from build123d import *

# Parameters (mm, degrees)
F0_W     = 762
F0_H     = 152.4
F1_DEPTH = 304.8
F2_T     = -25.4
F3_R     = 25.4
F4_DEPTH = 381
F5_R     = 12.7


with BuildPart() as f1:
    # F0 (on Front) → F1 (new body, symmetric)
    with BuildSketch(Plane.XZ):
        with Locations((0, 457.2)):
            Rectangle(F0_W, F0_H)
    extrude(amount=F1_DEPTH, both=True)

    # F2
    f2_openings = [f1.faces().sort_by_distance(p)[0] for p in [
        (0, -304.8, 457.2),
    ]]
    offset(amount=F2_T, openings=f2_openings)

    # F3 (on Top) → F4 (join, symmetric)
    with BuildSketch(Plane.XY):
        with Locations((-355.6, 279.4)):
            Circle(F3_R)
        with Locations((355.6, 279.4)):
            Circle(F3_R)
        with Locations((355.6, -279.4)):
            Circle(F3_R)
        with Locations((-355.6, -279.4)):
            Circle(F3_R)
    extrude(amount=F4_DEPTH, both=True)

    # F5
    f5_edges = [f1.edges().sort_by_distance(p)[0] for p in [
        (-381, 279.4, -381),
        (-381, -279.4, -381),
        (330.2, -279.4, -381),
        (330.2, 279.4, -381),
    ]]
    fillet(f5_edges, radius=F5_R)


solid = f1.part
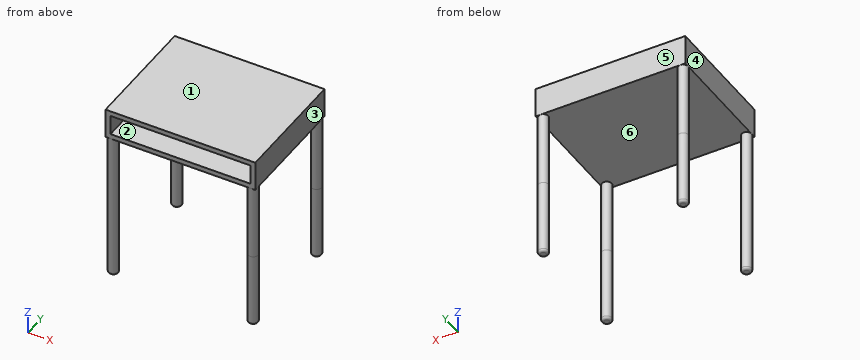
Check sheet for the modelled part. Datum: model origin and axes. Units: mm. Face numbers are marked on the shaded views. A direction names the side the tool comes from. Round coordinates to 2 decimals unless told otherwise and drop trailing zeros. Write each loop counter-clockwise with the first axis right and the second up, starting at its lowest first coordinate (ties: lowest second). Pieces come first, ordered by that corner, then holes. Notation, with made-up numbers: (-13.75, 32.25) - (34.25, 32.25) arc R14 ccw to (34.25, 37.25) - close; hole circle Ø3 at (-30.75, 49). An arc over 180 degrees is marked (long way). Return JSON: item names as keys, results as strings.
Q1. Cross-section at A-A (y = 93). Record the boundary of the cut face in (x, z).
Returned:
{"outline": "(-381, 381) - (381, 381) - (381, 533.4) - (-381, 533.4) - close; hole (-355.6, 406.4) - (355.6, 406.4) - (355.6, 508) - (-355.6, 508) - close"}
Q2. Depth check by flat-ended pin: P1, Ø7.5, axis at x = 373.5, y = -290, coming from the -Z side; P2, Ø3, axis at x = -59.5, y = -79, coming from the -Z side. Enter the tip coordinate at first touch or a pass-through.
Returned:
{"P1": "stops at z = -380.23", "P2": "stops at z = 381"}
Q3. Access from +Z, -Z, +X, -X, +Y, -Y to the whole of each face (thin tool, end or side, straight path). Record for the marked faces 5 and 6.
Returned:
{"face 5": "+Z, -Z, +X, -X, +Y", "face 6": "-Z"}
Q4. Cross-section at C-C (x = 75). Record the boundary of the cut face in (y, z), then the cut area to 3 significant figures.
Returned:
{"outline": "(-304.8, 381) - (304.8, 381) - (304.8, 533.4) - (-304.8, 533.4) - (-304.8, 508) - (279.4, 508) - (279.4, 406.4) - (-304.8, 406.4) - close", "area": "33,500 mm²"}
Q5. Scan lines: L1, parallel to Z at x = 142, y = 174.5; L2, parallel to X at y = -273, z = 452. Record each from-to range of solid material in increasing order. Write a range as from..to.
Returned:
{"L1": "z = 381..406.4, 508..533.4", "L2": "x = -381..-355.6, 355.6..381"}
Q6. Draft check along X on the marked faces 1, 2, 3 and 4. Enter one of: released by +X, released by -X, zero draft, split by the parting line, or undercut.
Returned:
{"face 1": "zero draft", "face 2": "undercut", "face 3": "released by +X", "face 4": "released by -X"}
Q7. Cross-section at B-B (z = -199). Record the boundary of the cut face in (x, y), then the cut area to 3 significant figures.
Returned:
{"outline": "circle Ø50.8 at (-355.6, -279.4); circle Ø50.8 at (-355.6, 279.4); circle Ø50.8 at (355.6, -279.4); circle Ø50.8 at (355.6, 279.4)", "area": "8,110 mm²"}
